Geometry check sheet. Reference: the model listing, model coordinates, mm. Face numbers are marked on the shaded views. A direction names the side the tool comes from. Coordinates: 2 decimals unless noted, no trailing zeros. Write each loop counter-clockwise with the first axis right and the second up, starting at its lowest first coordinate (ties: lowest second). Pieces come first, ordered by that corner, then holes. Notation, with made-up numbers: (21.5, -31) -> (75.5, -31) arc R16 ccw to (75.5, -3) -> close; hole circle Ø1 at (72.5, -1). An arc over 180 degrees is marked (long way). Answer as CSV lines item,"result".
```python
from build123d import *

# Parameters (mm, degrees)
SKETCH003_R      = 1.6
SKETCH003_R_2    = 1.7
EXTRUDE003_DEPTH = 10
SKETCH002_R      = 4
SKETCH002_R_2    = 2.5
SKETCH002_R_3    = 2
EXTRUDE002_DEPTH = 60
SKETCH001_W      = 79.47419
SKETCH001_H      = 9.458714
SKETCH001_W_2    = 5
EXTRUDE001_DEPTH = 40
EXTRUDE_DEPTH    = 110
FILLET_R         = 4
FILLET001_R      = 4


with BuildPart() as extrude003:
    # Sketch003 → Extrude003 (new body)
    with BuildSketch(Plane.XY):
        with Locations((5, 22)):
            Circle(SKETCH003_R)
        with Locations((49, 22)):
            Circle(SKETCH003_R)
        with Locations((61, 22)):
            Circle(SKETCH003_R)
        with Locations((105, 22)):
            Circle(SKETCH003_R)
        with Locations((81, 15)):
            Circle(SKETCH003_R_2)
        with Locations((106, 15)):
            Circle(SKETCH003_R_2)
    extrude(amount=EXTRUDE003_DEPTH)


with BuildPart() as fusion001:
    # Part__Mirroring001: instance of Extrude003
    add(extrude003.part.mirror(Plane(origin=(0, 0, 0), x_dir=(1, 0, 0), z_dir=(0, 1, 0))))

    # Fusion001: union Extrude003
    add(extrude003.part)


with BuildPart() as extrude002:
    # Sketch002 → Extrude002 (new body, symmetric)
    with BuildSketch(Plane.XZ):
        with Locations((11.1, 17.3)):
            Circle(SKETCH002_R)
        with Locations((22.1, 17.3)):
            Circle(SKETCH002_R_2)
        with Locations((31, 8.6)):
            Circle(SKETCH002_R_3)
        with Locations((31, 26)):
            Circle(SKETCH002_R_3)
    extrude(amount=EXTRUDE002_DEPTH, both=True)


with BuildPart() as extrude001:
    # Sketch001 → Extrude001 (new body)
    with BuildSketch(Plane.XY):
        with Locations((74.737095, 31.729357)):
            Rectangle(SKETCH001_W, SKETCH001_H)
        with Locations((2.5, 31.729357)):
            Rectangle(SKETCH001_W_2, SKETCH001_H)
    extrude(amount=EXTRUDE001_DEPTH)


with BuildPart() as part_mirroring:
    # Part__Mirroring: instance of Extrude001
    add(extrude001.part.mirror(Plane(origin=(0, 0, 0), x_dir=(1, 0, 0), z_dir=(0, 1, 0))))


with BuildPart() as fusion:
    # Fusion base: copy of Extrude001
    add(extrude001.part)

    # Fusion: union Part__Mirroring
    add(part_mirroring.part)


with BuildPart() as fillet001:
    # Sketch → Extrude (new body)
    with BuildSketch(Plane.YZ):
        with BuildLine():
            Line((-33, 30), (-33, 3))
            ThreePointArc((-33, 3), (-32.12132, 0.87868), (-30, 0))
            Line((-30, 0), (30, 0))
            ThreePointArc((30, 0), (32.12132, 0.87868), (33, 3))
            Line((33, 3), (33, 30))
            Line((33, 30), (31, 30))
            Line((31, 30), (31, 3))
            ThreePointArc((30, 2), (30.707107, 2.292893), (31, 3))
            Line((30, 2), (-30, 2))
            ThreePointArc((-31, 3), (-30.707107, 2.292893), (-30, 2))
            Line((-31, 3), (-31, 30))
            Line((-31, 30), (-33, 30))
        make_face()
    extrude(amount=EXTRUDE_DEPTH)

    # Cut: cut Fusion
    add(fusion.part, mode=Mode.SUBTRACT)

    # Cut001: cut Extrude002
    add(extrude002.part, mode=Mode.SUBTRACT)

    # Cut002: cut Fusion001
    add(fusion001.part, mode=Mode.SUBTRACT)

    # Fillet
    fillet_edges = [fillet001.edges().sort_by_distance(p)[0] for p in [
        (0, -27, 1),
        (110, -27, 1),
        (0, 27, 1),
        (110, 27, 1),
    ]]
    fillet(fillet_edges, radius=FILLET_R)

    # Fillet001
    fillet001_edges = [fillet001.edges().sort_by_distance(p)[0] for p in [
        (5, -32, 30),
        (35, -32, 30),
        (5, 32, 30),
        (35, 32, 30),
    ]]
    fillet(fillet001_edges, radius=FILLET001_R)


solid = fillet001.part
```
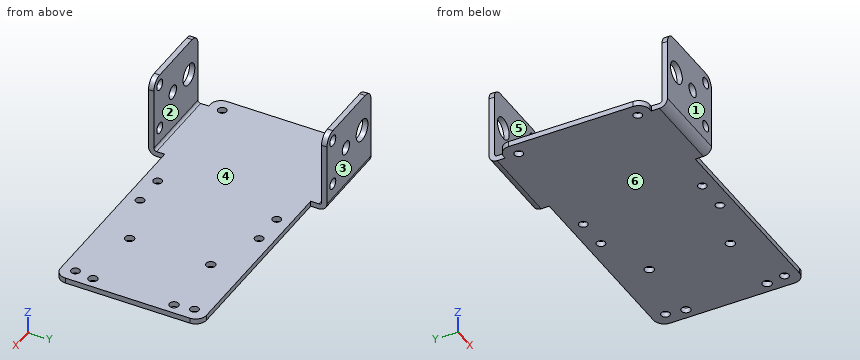
Item 1: Thickness scan on probe 1 along X at (y, z) = (-22, 1.5); probe 2 along X at (y, z) = (-32.25, 17.3); probe 3 along Y at (x, z) = (49, 1.35). Record the ranges inside material, lowest first.
Responses:
probe 1,"x = 0 to 3.4, 6.6 to 47.4, 50.6 to 59.4, 62.6 to 103.4, 106.6 to 110"
probe 2,"x = 5 to 7.1, 15.1 to 19.6, 24.6 to 35"
probe 3,"y = -27 to -23.6, -20.4 to 20.4, 23.6 to 27"
Item 2: Cross-section at D-D, the plane z = 17.3. Record the cut outline in (x, y), plus the area to 3 significant figures.
Responses:
outline,"(5, -33) -> (7.1, -33) -> (7.1, -31) -> (5, -31) -> close; (5, 31) -> (7.1, 31) -> (7.1, 33) -> (5, 33) -> close; (15.1, -33) -> (19.6, -33) -> (19.6, -31) -> (15.1, -31) -> close; (15.1, 31) -> (19.6, 31) -> (19.6, 33) -> (15.1, 33) -> close; (24.6, -33) -> (35, -33) -> (35, -31) -> (24.6, -31) -> close; (24.6, 31) -> (35, 31) -> (35, 33) -> (24.6, 33) -> close"
area,"68.0 mm2"
Item 3: Cross-section at C-C, the plane y = -15. Record the cut outline in (x, z), plus the area to 3 significant figures.
Responses:
outline,"(0, 0) -> (79.3, 0) -> (79.3, 2) -> (0, 2) -> close; (82.7, 0) -> (104.3, 0) -> (104.3, 2) -> (82.7, 2) -> close; (107.7, 0) -> (110, 0) -> (110, 2) -> (107.7, 2) -> close"
area,"206 mm2"
Item 4: Set-up check for the marked faces 1 and 2: record each of +Z, -Z, +X, -X, +Y, -Y from which the full face is reachable in a straight line by a thin tool's end or side.
Responses:
face 1,"+Z, -Z, +X, -X, -Y"
face 2,"+Z, +X, -X"
Item 5: Depth check by flat-ended pin: pin 1 Ø2.5 at (x, y) = (105, 22) entering from +Z; pin 2 Ø2 at (x, z) = (59, 1) entering from +Y; pin 3 Ø2 at (x, y) = (16, 17) entering from +Z; pin 4 Ø0.8 at (x, z) = (4.5, 1) entering from -Y. Enter the tip coordinate at first touch or a pass-through.
Responses:
pin 1,"passes through"
pin 2,"stops at y = 27"
pin 3,"stops at z = 2"
pin 4,"stops at y = -27"
Item 6: Cross-section at A-A, the plane x = 49. Record the cut outline in (y, z).
Responses:
outline,"(-27, 0) -> (-23.6, 0) -> (-23.6, 2) -> (-27, 2) -> close; (-20.4, 0) -> (20.4, 0) -> (20.4, 2) -> (-20.4, 2) -> close; (23.6, 0) -> (27, 0) -> (27, 2) -> (23.6, 2) -> close"
Item 7: Release check for a two-part mould opening along Y. For the marked faces 3, 4, 5 and 6 record: +Y half, -Y half, draft (parallel to the pull), parting line (faces both ways), or undercut.
Responses:
face 3,"+Y half"
face 4,"undercut"
face 5,"undercut"
face 6,"draft"
Item 8: Cross-section at B-B, the plane z = 8.6. Record the cut outline in (x, y), plus the area to 3 significant figures.
Responses:
outline,"(5, -33) -> (29, -33) -> (29, -31) -> (5, -31) -> close; (5, 31) -> (29, 31) -> (29, 33) -> (5, 33) -> close; (33, -33) -> (35, -33) -> (35, -31) -> (33, -31) -> close; (33, 31) -> (35, 31) -> (35, 33) -> (33, 33) -> close"
area,"104 mm2"
